```python
from build123d import *

# Parameters (mm, degrees)
SKICA1_W                    = 67
SKICA1_H                    = 50
P_IDAT_VYSUNUT_M1_DEPTH     = 3
ODEBRAT_VYSUNUT_M1_DEPTH    = 1
SKICA3_W                    = 8
SKICA3_H                    = 8
ODEBRAT_VYSUNUT_M2_DEPTH    = 4
VYSUNOUT_TENKOST_NN_1_DEPTH = 1
VYSUNOUT_TENKOST_NN_2_DEPTH = 5
SKICA6_W                    = 12
SKICA6_H                    = 4
ODEBRAT_VYSUNUT_M3_DEPTH    = 4
ODEBRAT_VYSUNUT_M5_DEPTH    = 1
P_IDAT_START                = -1
P_IDAT_VYSUNUT_M3_DEPTH     = 1
ODEBRAT_VYSUNUT_M6_DEPTH    = 1
SKICA10_W                   = 1.6
SKICA10_H                   = 2.4
P_IDAT_VYSUNUT_M4_DEPTH     = 1


with BuildPart() as part:
    # Skica1 → Přidat vysunutím1 (new body)
    with BuildSketch(Plane.XY):
        Rectangle(SKICA1_W, SKICA1_H)
    extrude(amount=P_IDAT_VYSUNUT_M1_DEPTH)

    # Skica2 → Odebrat vysunutím1 (cut)
    with BuildSketch(Plane.XY.offset(3)):
        Polygon((-25.5, -22), (-30.5, -17), (-30.5, 17), (-25.5, 22), (25.5, 22), (30.5, 17), (30.5, -17), (25.5, -22), align=None)
    extrude(amount=-ODEBRAT_VYSUNUT_M1_DEPTH, mode=Mode.SUBTRACT)

    # Skica3 → Odebrat vysunutím2 (cut, through all)
    with BuildSketch(Plane(origin=(0, 0, 0), x_dir=(-1, 0, 0), z_dir=(0, 0, -1))):
        with Locations((20, -3)):
            Rectangle(SKICA3_W, SKICA3_H)
        with Locations((-20, -3)):
            Rectangle(SKICA3_W, SKICA3_H)
        Polygon((25.5, -25), (-25.5, -25), (-25.5, -12), (-12, -12), (-12, 15), (12, 15), (12, -12), (25.5, -12), align=None)
    extrude(amount=-ODEBRAT_VYSUNUT_M2_DEPTH, mode=Mode.SUBTRACT)

    # Skica4 → Vysunout tenkostěnný1 (add)
    with BuildSketch(Plane.XY.offset(2)):
        Polygon((-12, -12), (-12, 15), (12, 15), (12, -12), (13, -12), (13, 16), (-13, 16), (-13, -12), align=None)
    extrude(amount=VYSUNOUT_TENKOST_NN_1_DEPTH)

    # Skica5 → Vysunout tenkostěnný2 (add)
    with BuildSketch(Plane(origin=(0, 0, 0), x_dir=(-1, 0, 0), z_dir=(0, 0, -1))):
        Polygon((-25.5, -25), (-33.5, -25), (-33.5, 25), (33.5, 25), (33.5, -25), (25.5, -25), (25.5, -26), (34.5, -26), (34.5, 26), (-34.5, 26), (-34.5, -26), (-25.5, -26), align=None)
    extrude(amount=-VYSUNOUT_TENKOST_NN_2_DEPTH)

    # Skica6 → Odebrat vysunutím3 (cut, through all)
    with BuildSketch(Plane.XY.offset(2)):
        with Locations((0, 24)):
            Rectangle(SKICA6_W, SKICA6_H)
    extrude(amount=ODEBRAT_VYSUNUT_M3_DEPTH, mode=Mode.SUBTRACT)

    # Skica7 → Odebrat vysunutím5 (cut)
    with BuildSketch(Plane(origin=(0, 0, 0), x_dir=(-1, 0, 0), z_dir=(0, 0, -1))):
        Polygon((-32.44, 14.540476732), (-23.459523268, 23.94), (-14.06, 14.959523268), (-23.040476732, 5.56), align=None)
        Polygon((14.06, 14.959523268), (23.040476732, 5.56), (32.44, 14.540476732), (23.459523268, 23.94), align=None)
    extrude(amount=-ODEBRAT_VYSUNUT_M5_DEPTH, mode=Mode.SUBTRACT)

    # Skica8 → Přidat vysunutím3 (add)
    with BuildSketch(Plane(origin=(0, 0, 0), x_dir=(-1, 0, 0), z_dir=(0, 0, -1)).offset(P_IDAT_START)):
        Polygon((-29.266904741, 14.966465555), (-27.459304113, 13.239450799), (-25.766904741, 15.010820822), align=None)
        Polygon((-23.626799477, 17.250787567), (-21.932856893, 19.023772811), (-23.740457522, 20.750787567), align=None)
        Polygon((-24.551025932, 9.769304113), (-26.358626561, 11.496318869), (-25.667820659, 12.21935912), (-23.940805902, 12.21935912), (-23.940805902, 14.026959749), (-22.559194098, 15.473040251), (-20.832179341, 15.473040251), (-20.832179341, 17.28064088), (-20.141373439, 18.003681131), (-18.333772811, 16.276666375), (-20.751593469, 13.746025495), (-22.304085189, 13.84625566), (-22.133205274, 12.299944993), align=None)
        Polygon((27.459304113, 13.239450799), (25.766904741, 15.010820822), (29.266904741, 14.966465555), align=None)
        Polygon((23.626799477, 17.250787567), (21.932856893, 19.023772811), (23.740457522, 20.750787567), align=None)
        Polygon((23.940805902, 14.026959749), (22.559194098, 15.473040251), (20.832179341, 15.473040251), (20.832179341, 17.28064088), (20.141373439, 18.003681131), (18.333772811, 16.276666375), (20.751593469, 13.746025495), (22.304085189, 13.84625566), (22.133205274, 12.299944993), (24.551025932, 9.769304113), (26.358626561, 11.496318869), (25.667820659, 12.21935912), (23.940805902, 12.21935912), align=None)
    extrude(amount=P_IDAT_VYSUNUT_M3_DEPTH)

    # Skica9 → Odebrat vysunutím6 (cut)
    with BuildSketch(Plane(origin=(0, 0, 0), x_dir=(-1, 0, 0), z_dir=(0, 0, -1))):
        Polygon((-10.3, 23.3), (-7.1, 23.3), (-7.1, 22.5), (-6.3, 22.5), (-6.3, 21.7), (-7.9, 21.7), (-7.9, 22.5), (-9.5, 22.5), (-9.5, 18.5), (-7.9, 18.5), (-7.9, 19.3), (-8.7, 19.3), (-8.7, 20.1), (-6.3, 20.1), (-6.3, 18.5), (-7.1, 18.5), (-7.1, 17.7), (-10.3, 17.7), (-10.3, 18.5), (-11.1, 18.5), (-11.1, 22.5), (-10.3, 22.5), align=None)
        Polygon((-5.3, 23.3), (-1.3, 23.3), (-1.3, 22.3), (-4, 22.3), (-4, 21), (-2.4, 21), (-2.4, 20), (-4, 20), (-4, 18.7), (-1.3, 18.7), (-1.3, 17.7), (-5.3, 17.7), align=None)
        Polygon((-0.3, 23.3), (1.3, 23.3), (1.3, 22.5), (2.1, 22.5), (2.1, 21.7), (2.9, 21.7), (2.9, 22.5), (3.7, 22.5), (3.7, 23.3), (5.3, 23.3), (5.3, 17.7), (3.7, 17.7), (3.7, 20.7), (2.9, 20.7), (2.9, 19.9), (2.1, 19.9), (2.1, 20.7), (1.3, 20.7), (1.3, 17.7), (-0.3, 17.7), align=None)
        Polygon((7.1, 23.3), (10.3, 23.3), (10.3, 22.5), (11.1, 22.5), (11.1, 18.5), (10.3, 18.5), (10.3, 17.7), (7.1, 17.7), (7.1, 18.5), (6.3, 18.5), (6.3, 22.5), (7.1, 22.5), align=None)
    extrude(amount=-ODEBRAT_VYSUNUT_M6_DEPTH, mode=Mode.SUBTRACT)

    # Skica10 → Přidat vysunutím4 (add)
    with BuildSketch(Plane(origin=(0, 0, 1), x_dir=(-1, 0, 0), z_dir=(0, 0, -1))):
        with Locations((8.7, 20.5)):
            Rectangle(SKICA10_W, SKICA10_H)
    extrude(amount=P_IDAT_VYSUNUT_M4_DEPTH)


solid = part.part
```
The listing builds one solid part. Answer for the finished solid, in the listing's coordinates (mm). A direction names the side the tool comes from. Coordinates: 2 decimals unless noted, no trailing zeros. Write each loop counter-clockwise with the first axis right and the second up, starting at its lowest first coordinate (ties: lowest second). Pieces come first, ordered by that corner, then holes. Notation, with made-up numbers: (-10, -6) - (26, -6) arc R20 cw to (26, 14) - close; hole circle Ø7 at (27.25, 56). An arc over 180 degrees is marked (long way). Return JSON: item names as keys, results as strings. Group by question number.
Q1. Flat-ended cylindrical pins translate along their axes: pin 1 Ø5 at (x, y) = (-13, 4) entering from +Z; pin 2 Ø1.6 at (x, z) = (18, 1) entering from -Y; pin 3 Ø1.5 at (x, y) = (15.5, -8.5) entering from +Z. Find the tip coordinate at first contact, or state that the pin passes through.
Q2. The part is cut by section B-B on x = -17. Write down the section's boundary in (y, z), and give its area (3 significant figures).
Q3. For a pull along Y with two mould halves and no side action, classify faces 1 (the flat face through (0, 26, 1)), 2 (the flat face through (-27.674, 9.987, 0.493)), 3 (the flat face through (-6, 24.4, 2.8)) as +Y half, -Y half, draft (parallel to the pull), parting line (faces both ways), or undercut.
Q4. Find the intervals of material crossed by line 1 along X through (y, z) = (6.5, 2.5); line 2 along X through (y, z) = (-4, 1.05); line 3 along X through (y, z) = (5, 1.95), in increasing order. Write a range as [from, to].
Q5. The part is cut by section C-C on x = -0.5. Write down the section's boundary in (y, z), and give its area (3 significant figures).
Q6. Which of the six approach directions +Z, -Z, +X, -X, +Y, -Y give full straight-line access (tool end or side, diameter ignored) to faces 4 (the flat face through (-19.526, 15.029, 0.507)), 5 (the flat face through (-12, 1, 1)), 6 (the flat face through (-0.1, 15.5, 3))?
Q7. The part is cut by section A-A on y = -13. Write down the section's boundary in (x, z), and give its area (3 significant figures).
Evaluation:
{
 "1": {"pin 1": "stops at z = 3", "pin 2": "stops at y = -12", "pin 3": "stops at z = 2"},
 "2": {"outline": "(-12, 0) - (-7, 0) - (-7, 2) - (-12, 2) - close; (1, 0) - (11.88, 0) - (11.88, 1) - (17.77, 1) - (17.77, 0) - (26, 0) - (26, 5) - (25, 5) - (25, 3) - (22, 3) - (22, 2) - (1, 2) - close", "area": "60.1 mm2"},
 "3": {"face 1": "+Y half", "face 2": "undercut", "face 3": "draft"},
 "4": {"line 1": "x = [-34.5, -30.5], [-13, -12], [12, 13], [30.5, 34.5]", "line 2": "x = [-34.5, -24], [-16, -12], [12, 16], [24, 34.5]", "line 3": "x = [-34.5, -12], [12, 34.5]"},
 "5": {"outline": "(15, 0) - (17.7, 0) - (17.7, 1) - (23.3, 1) - (23.3, 0) - (26, 0) - (26, 2) - (16, 2) - (16, 3) - (15, 3) - close", "area": "17.4 mm2"},
 "6": {"face 4": "-Z", "face 5": "+Z, -Z, -Y", "face 6": "+Z, -Y"},
 "7": {"outline": "(-34.5, 0) - (-25.5, 0) - (-25.5, 2) - (-30.5, 2) - (-30.5, 3) - (-33.5, 3) - (-33.5, 5) - (-34.5, 5) - close; (25.5, 0) - (34.5, 0) - (34.5, 5) - (33.5, 5) - (33.5, 3) - (30.5, 3) - (30.5, 2) - (25.5, 2) - close", "area": "48.0 mm2"}
}
